```python
from build123d import *

# Parameters (mm, degrees)
BOSS_EXTRUDE1_DEPTH             = 76.2
BOSS_EXTRUDE1_DEPTH_BACK        = 76.2
CUT_EXTRUDE1_DEPTH              = 136.619651209
CUT_EXTRUDE1_DEPTH_BACK         = 136.619651209
FILLET1_R                       = 3.81
SHELL1_START                    = -44.45
SHELL1_DEPTH                    = 88.773
SHELL1_START_2                  = -73.025
SHELL1_2_DEPTH                  = 130.048
SKETCH14_R                      = 2.032
CUT_EXTRUDE8_DEPTH              = 156.372005628
BOSS_EXTRUDE4_REACH             = 137.201
SKETCH15_R                      = 1.5875
BOSS_EXTRUDE4_DIRECTION_2_REACH = 137.201


# Read off the part's stored shape, not the designer's step: Shell1
with BuildPart() as part:
    # Sketch1 → Boss-Extrude1 (new, two sides: drawn at the far end of the back side and taken through both)
    with BuildSketch(Plane.XY.offset(-BOSS_EXTRUDE1_DEPTH_BACK)):
        with BuildLine():
            Line((-6.335258536, -105.245804705), (-12.685258536, -3.645804705))
            ThreePointArc((-12.685258536, -3.645804705), (0.014741464, 8.866413132), (12.714741464, -3.645804705))
            Line((12.714741464, -3.645804705), (6.364741464, -105.245804705))
            ThreePointArc((6.364741464, -105.245804705), (0.014741464, -111.465623147), (-6.335258536, -105.245804705))
        make_face()
    extrude(amount=BOSS_EXTRUDE1_DEPTH + BOSS_EXTRUDE1_DEPTH_BACK)

    # Sketch4 → Cut-Extrude1 (cut, two sides: drawn at the far end of the back side and taken through both)
    with BuildSketch(Plane(origin=(0, 0, 0), x_dir=(0, 0, -1), z_dir=(1, 0, 0)).offset(-CUT_EXTRUDE1_DEPTH_BACK)):
        Polygon((-47.498, -73.524605007), (-47.498, -51.299605007), (47.625, -51.299605007), (47.625, -73.524605007), (76.2, -73.524605007), (76.2, 8.866413132), (-76.2, 8.866413132), (-76.2, -28.682279346), (-76.2, -111.465623147), (-60.198, -111.465623147), (-60.198, -73.524605007), align=None)
    extrude(amount=CUT_EXTRUDE1_DEPTH + CUT_EXTRUDE1_DEPTH_BACK, mode=Mode.SUBTRACT)

    # Fillet1
    fillet1_edges = [part.edges().sort_by_distance(p)[0] for p in [
        (8.347316445, -73.524605007, 53.848),
        (9.736378945, -51.299605007, -0.0635),
        (-9.706896017, -51.299605007, -0.0635),
        (-8.317833517, -73.524605007, 53.848),
        (-8.317833517, -73.524605007, -61.9125),
        (8.347316445, -73.524605007, -61.9125),
    ]]
    fillet(fillet1_edges, radius=FILLET1_R)

    # Shell1 outline → Shell1 (cut)
    with BuildSketch(Plane.XY.offset(SHELL1_START)):
        with BuildLine():
            ThreePointArc((-3.161602106, -105.125185529), (0.014741465, -108.290623147), (3.191085035, -105.125185529))
            Line((3.191085035, -105.125185529), (6.314583179, -55.149215219))
            ThreePointArc((6.314583179, -55.149215219), (6.143625088, -54.674822007), (5.680819792, -54.474605007))
            Line((5.680819792, -54.474605007), (-5.651336863, -54.474605007))
            ThreePointArc((-5.651336863, -54.474605007), (-6.114142159, -54.674822006), (-6.285100251, -55.149215219))
            Line((-6.285100251, -55.149215219), (-3.161602106, -105.125185529))
        make_face()
    extrude(amount=SHELL1_DEPTH, mode=Mode.SUBTRACT)

    # Shell1 2 outline → Shell1 2 (cut)
    with BuildSketch(Plane.XY.offset(SHELL1_START_2)):
        with BuildLine():
            Line((-4.896037751, -77.374215219), (-3.161602106, -105.125185529))
            ThreePointArc((-3.161602106, -105.125185529), (0.014741465, -108.290623147), (3.191085035, -105.125185529))
            Line((3.191085035, -105.125185529), (4.925520679, -77.374215219))
            ThreePointArc((4.925520679, -77.374215219), (4.754562588, -76.899822007), (4.291757292, -76.699605007))
            Line((4.291757292, -76.699605007), (-4.262274363, -76.699605007))
            ThreePointArc((-4.262274363, -76.699605007), (-4.725079659, -76.899822006), (-4.896037751, -77.374215219))
        make_face()
    extrude(amount=SHELL1_2_DEPTH, mode=Mode.SUBTRACT)

    # Sketch14 → Cut-Extrude8 (cut, through all)
    with BuildSketch(Plane(origin=(0, 0, -47.625), x_dir=(-1, 0, 0), z_dir=(0, 0, -1))):
        with Locations((-0.014741464, -61.459605007)):
            Circle(SKETCH14_R)
    extrude(amount=-CUT_EXTRUDE8_DEPTH, mode=Mode.SUBTRACT)

    # Boss-Extrude4: up to this plane
    boss_extrude4_end = Plane(origin=(3.195924528, -105.047753647, -76.2), z_dir=(0.9980525784828886, -0.062378286155180485, 0))
    # Sketch15 → Boss-Extrude4 (add, up to the surface)
    with BuildSketch(Plane(origin=(3.191103822, -0.502900096, 0), x_dir=(0, 0, -1), z_dir=(1, 0, 0)), mode=Mode.PRIVATE) as boss_extrude4_sk1:
        with Locations(Location((-9.398, -66.274366182, 0), (0, 0, 270))):
            Circle(SKETCH15_R)
    boss_extrude4_tool1 = split(extrude(boss_extrude4_sk1.sketch, amount=BOSS_EXTRUDE4_REACH, mode=Mode.PRIVATE), bisect_by=boss_extrude4_end, keep=Keep.BOTH, mode=Mode.PRIVATE)
    add(boss_extrude4_tool1.solids().sort_by_distance((3.191104, -66.777266, 9.398))[0])
    # Sketch15 → Boss-Extrude4 (add, up to the surface)
    with BuildSketch(Plane(origin=(3.191103822, -0.502900096, 0), x_dir=(0, 0, -1), z_dir=(1, 0, 0)), mode=Mode.PRIVATE) as boss_extrude4_sk2:
        with Locations(Location((26.868345804, -77.595887652, 0), (0, 0, 270))):
            Circle(SKETCH15_R)
    boss_extrude4_tool2 = split(extrude(boss_extrude4_sk2.sketch, amount=BOSS_EXTRUDE4_REACH, mode=Mode.PRIVATE), bisect_by=boss_extrude4_end, keep=Keep.BOTH, mode=Mode.PRIVATE)
    add(boss_extrude4_tool2.solids().sort_by_distance((3.191104, -78.098788, -26.868346))[0])
    # Sketch15 → Boss-Extrude4 (add, up to the surface)
    with BuildSketch(Plane(origin=(3.191103822, -0.502900096, 0), x_dir=(0, 0, -1), z_dir=(1, 0, 0)), mode=Mode.PRIVATE) as boss_extrude4_sk3:
        with Locations(Location((-22.098, -96.55076585, 0), (0, 0, 270))):
            Circle(SKETCH15_R)
    boss_extrude4_tool3 = split(extrude(boss_extrude4_sk3.sketch, amount=BOSS_EXTRUDE4_REACH, mode=Mode.PRIVATE), bisect_by=boss_extrude4_end, keep=Keep.BOTH, mode=Mode.PRIVATE)
    add(boss_extrude4_tool3.solids().sort_by_distance((3.191104, -97.053666, 22.098))[0])
    # Sketch15 → Boss-Extrude4 (add, up to the surface)
    with BuildSketch(Plane(origin=(3.191103822, -0.502900096, 0), x_dir=(0, 0, -1), z_dir=(1, 0, 0)), mode=Mode.PRIVATE) as boss_extrude4_sk4:
        with Locations(Location((16.002, -96.55076585, 0), (0, 0, 270))):
            Circle(SKETCH15_R)
    boss_extrude4_tool4 = split(extrude(boss_extrude4_sk4.sketch, amount=BOSS_EXTRUDE4_REACH, mode=Mode.PRIVATE), bisect_by=boss_extrude4_end, keep=Keep.BOTH, mode=Mode.PRIVATE)
    add(boss_extrude4_tool4.solids().sort_by_distance((3.191104, -97.053666, -16.002))[0])
    # Sketch15 → Boss-Extrude4 (add, up to the surface)
    with BuildSketch(Plane(origin=(3.191103822, -0.502900096, 0), x_dir=(0, 0, -1), z_dir=(1, 0, 0)), mode=Mode.PRIVATE) as boss_extrude4_sk5:
        with Locations(Location((54.102, -96.55076585, 0), (0, 0, 270))):
            Circle(SKETCH15_R)
    boss_extrude4_tool5 = split(extrude(boss_extrude4_sk5.sketch, amount=BOSS_EXTRUDE4_REACH, mode=Mode.PRIVATE), bisect_by=boss_extrude4_end, keep=Keep.BOTH, mode=Mode.PRIVATE)
    add(boss_extrude4_tool5.solids().sort_by_distance((3.191104, -97.053666, -54.102))[0])

    # Boss-Extrude4 direction 2: up to this plane
    boss_extrude4_direction_2_end = Plane(origin=(-3.166441599, -105.047753647, -76.2), z_dir=(-0.9980525784828886, -0.0623782861551806, 0))
    # Sketch15 → Boss-Extrude4 direction 2 (add, up to the surface)
    with BuildSketch(Plane(origin=(3.191103822, -0.502900096, 0), x_dir=(0, 0, -1), z_dir=(1, 0, 0)), mode=Mode.PRIVATE) as boss_extrude4_direction_2_sk1:
        with Locations(Location((-9.398, -66.274366182, 0), (0, 0, 270))):
            Circle(SKETCH15_R)
    boss_extrude4_direction_2_tool1 = split(extrude(boss_extrude4_direction_2_sk1.sketch, amount=-BOSS_EXTRUDE4_DIRECTION_2_REACH, mode=Mode.PRIVATE), bisect_by=boss_extrude4_direction_2_end, keep=Keep.BOTH, mode=Mode.PRIVATE)
    add(boss_extrude4_direction_2_tool1.solids().sort_by_distance((3.191104, -66.777266, 9.398))[0])
    # Sketch15 → Boss-Extrude4 direction 2 (add, up to the surface)
    with BuildSketch(Plane(origin=(3.191103822, -0.502900096, 0), x_dir=(0, 0, -1), z_dir=(1, 0, 0)), mode=Mode.PRIVATE) as boss_extrude4_direction_2_sk2:
        with Locations(Location((26.868345804, -77.595887652, 0), (0, 0, 270))):
            Circle(SKETCH15_R)
    boss_extrude4_direction_2_tool2 = split(extrude(boss_extrude4_direction_2_sk2.sketch, amount=-BOSS_EXTRUDE4_DIRECTION_2_REACH, mode=Mode.PRIVATE), bisect_by=boss_extrude4_direction_2_end, keep=Keep.BOTH, mode=Mode.PRIVATE)
    add(boss_extrude4_direction_2_tool2.solids().sort_by_distance((3.191104, -78.098788, -26.868346))[0])
    # Sketch15 → Boss-Extrude4 direction 2 (add, up to the surface)
    with BuildSketch(Plane(origin=(3.191103822, -0.502900096, 0), x_dir=(0, 0, -1), z_dir=(1, 0, 0)), mode=Mode.PRIVATE) as boss_extrude4_direction_2_sk3:
        with Locations(Location((-22.098, -96.55076585, 0), (0, 0, 270))):
            Circle(SKETCH15_R)
    boss_extrude4_direction_2_tool3 = split(extrude(boss_extrude4_direction_2_sk3.sketch, amount=-BOSS_EXTRUDE4_DIRECTION_2_REACH, mode=Mode.PRIVATE), bisect_by=boss_extrude4_direction_2_end, keep=Keep.BOTH, mode=Mode.PRIVATE)
    add(boss_extrude4_direction_2_tool3.solids().sort_by_distance((3.191104, -97.053666, 22.098))[0])
    # Sketch15 → Boss-Extrude4 direction 2 (add, up to the surface)
    with BuildSketch(Plane(origin=(3.191103822, -0.502900096, 0), x_dir=(0, 0, -1), z_dir=(1, 0, 0)), mode=Mode.PRIVATE) as boss_extrude4_direction_2_sk4:
        with Locations(Location((16.002, -96.55076585, 0), (0, 0, 270))):
            Circle(SKETCH15_R)
    boss_extrude4_direction_2_tool4 = split(extrude(boss_extrude4_direction_2_sk4.sketch, amount=-BOSS_EXTRUDE4_DIRECTION_2_REACH, mode=Mode.PRIVATE), bisect_by=boss_extrude4_direction_2_end, keep=Keep.BOTH, mode=Mode.PRIVATE)
    add(boss_extrude4_direction_2_tool4.solids().sort_by_distance((3.191104, -97.053666, -16.002))[0])
    # Sketch15 → Boss-Extrude4 direction 2 (add, up to the surface)
    with BuildSketch(Plane(origin=(3.191103822, -0.502900096, 0), x_dir=(0, 0, -1), z_dir=(1, 0, 0)), mode=Mode.PRIVATE) as boss_extrude4_direction_2_sk5:
        with Locations(Location((54.102, -96.55076585, 0), (0, 0, 270))):
            Circle(SKETCH15_R)
    boss_extrude4_direction_2_tool5 = split(extrude(boss_extrude4_direction_2_sk5.sketch, amount=-BOSS_EXTRUDE4_DIRECTION_2_REACH, mode=Mode.PRIVATE), bisect_by=boss_extrude4_direction_2_end, keep=Keep.BOTH, mode=Mode.PRIVATE)
    add(boss_extrude4_direction_2_tool5.solids().sort_by_distance((3.191104, -97.053666, -54.102))[0])


solid = part.part
```
Model file for the job. Use its own axes, mm. A direction names the side the tool comes from. Give positions to 0.01 mm unless a question says otherwise; leave off trailing zeros. Loops run counter-clockwise (first coordinate to the right, second up) from the corner with the lowest first, then second, coordinate; pieces in that order, holes last. Notation, with made-up numbers: (87, 73.5) -> (115, 73.5) arc R18 cw to (115, 84.5) -> close; hole circle Ø4 at (22.5, -9.75). An arc over 180 degrees is marked (long way). Write each question's results on one line, items separated by ' | '.
(1) Probe line 1 along Z through (x, y) = (3, -58) (3 decimals); line 2 along Z through (x, y) = (0.25, -101.5) (3 decimals); line 3 along X through (y, z) = (-55, -41.5). List the from-to ranges inside material, lowest first.
Geometry results:
line 1: z = -47.625 to -44.45, 44.323 to 47.498 | line 2: z = -76.2 to -73.025, 57.023 to 60.198 | line 3: x = -9.46 to -6.28, 6.31 to 9.49
(2) Cut at C-C on y = -88. List the corners of the cut face in (x, z) (3 decimals).
Geometry results:
outline: (-7.413, -76.2) -> (7.443, -76.2) -> (7.443, 60.198) -> (-7.413, 60.198) -> close; hole (-4.232, -73.025) -> (4.261, -73.025) -> (4.261, 57.023) -> (-4.232, 57.023) -> close
(3) Cut at B-B on x = 0.5. Give the number of separate pieces and of enclosed holes in the cut face, and give its area (3 significant figures).
Geometry results:
separate pieces: 7 | enclosed holes: 0 | area: 1,220 mm²
(4) Cut at A-A on z = 13. List the corners of the cut face in (x, y) (3 decimals), and give its area (3 significant figures).
Geometry results:
outline: (-9.454, -55.347) -> (-6.335, -105.246) arc R6.351 ccw to (6.365, -105.246) -> (9.483, -55.347) arc R3.81 ccw to (5.681, -51.3) -> (-5.651, -51.3) arc R3.81 ccw to start; hole (-6.285, -55.149) -> (-3.162, -105.125) arc R3.176 ccw to (3.191, -105.125) -> (6.315, -55.149) arc R0.635 ccw to (5.681, -54.475) -> (-5.651, -54.475) arc R0.635 ccw to start | area: 424 mm²
(5) Tool access for faces 1 (the flat face through (0, -73.525, 54)), 2 (the flat face through (0, -51.3, 1)), 3 (the cylindrical face through (-0.05, -108.29, -8.91)): list every direction of +Z, -Z, +X, -X, +Y, -Y with a clear straight run to the whole face (end or side of a thin tool).
Geometry results:
face 1: +Z, +X, -X, +Y | face 2: +Z, -Z, +X, -X, +Y | face 3: none
(6) Pull direction Y, two halves, no side cores. Call faces 4 (the flat face through (0, -92, -73.025)), 5 (the cylindrical face through (0.455, -63.443, -46.06)), 6 (the flat face through (7.946, -79.947, -8.956)), 7 (the flat face through (0, -92, -76.2)): released by +Y, released by -Y, zero draft, split by the parting line, or undercut.
Geometry results:
face 4: undercut | face 5: undercut | face 6: released by -Y | face 7: zero draft
(7) Flat gauge pins, fed straight in: pin 1 Ø2.5 at (x, y) = (0.01, -61.46) entering from -Z; pin 2 Ø7 at (x, z) = (1.5, -60.5) entering from +Y; pin 3 Ø4 at (x, y) = (-1, -66.5) entering from +Z; pin 4 Ø3 at (x, z) = (-5, -17.5) entering from -Y. Where does each tip first touch, or does it go through?
Geometry results:
pin 1: passes through | pin 2: stops at y = -73.52 | pin 3: stops at z = 47.5 | pin 4: stops at y = -110.4
(8) Cut at D-D on z = -65.5. List the corners of the cut face in (x, y) (3 decimals).
Geometry results:
outline: (-8.065, -77.572) -> (-6.335, -105.246) arc R6.351 ccw to (6.365, -105.246) -> (8.094, -77.572) arc R3.81 ccw to (4.292, -73.525) -> (-4.262, -73.525) arc R3.81 ccw to start; hole (-4.896, -77.374) -> (-3.162, -105.125) arc R3.176 ccw to (3.191, -105.125) -> (4.926, -77.374) arc R0.635 ccw to (4.292, -76.7) -> (-4.262, -76.7) arc R0.635 ccw to start
